Autodesk Inventor part; units mm, degrees
ref_plane "YZ Plane" through (0, 0, 0) normal (1, 0, 0) x (0, 1, 0)
ref_plane "XZ Plane" through (0, 0, 0) normal (0, 1, 0) x (-1, 0, 0)
ref_plane "XY Plane" through (0, 0, 0) normal (0, 0, 1) x (1, 0, 0)
sketch "Sketch2" plane through (0, 0, 0) normal (1, 0, 0) x (0, 1, 0)
  line L0 (0, 0) -> (39, 0)
  line L1 (44, -5) -> (44, -5)
  line L2 (34, -5) -> (0, -5)
  line L3 (0, -5) -> (0, 0)
  line L4 (39, -10) -> (39, -43)
  line L5 (44, -48) -> (44, -5)
  line L6 (0, -53) -> (0, -48)
  line L7 (39, -53) -> (0, -53)
  line L8 (0, -53) -> (0, -48)
  line L9 (0, -48) -> (34, -48)
  arc A0 (44, -5) -> (39, 0) centre (39, -5) ccw
  arc A1 (34, -48) -> (39, -43) centre (34, -43) ccw
  arc A2 (39, -10) -> (34, -5) centre (34, -10) ccw
  arc A3 (39, -53) -> (44, -48) centre (39, -48) ccw
  point P0 (44, 0)
  point P1 (0, -2.5)
  point P2 (0, -53)
  dimension "d12" = 44
  dimension "d14" = 5
  dimension "d17" = 5
  dimension "d18" = 39
  dimension "d19" = 5
  dimension "d42" = 43
extrude "Extrusion2" add sketch "Sketch2" along normal blind 14.25
fillet "Fillet1" radius 4 4 edges at (14.25, 0, -2.5) (0, 0, -2.5) (14.25, 0, -50.5) (0, 0, -50.5)
sketch "Sketch3" plane through (0, 39, 0) normal (0, 0, 1) x (1, 0, 0)
  circle A0 centre (7.125, -33.3) radius 2.8
  line L0 (0, 0) -> (0, -35)
  line L1 (4, -39) -> (10.25, -39)
  point P0 (0, -39)
  point P1 (7.125, -39)
  dimension "d23" = 5.6
  dimension "d24" = 7.125
  dimension "d25" = 5.7
extrude "Extrusion3" cut sketch "Sketch3" against normal blind 11.4
sketch "Sketch7" plane through (0, 39, -43) normal (0, -1, 0) x (1, 0, 0)
  circle A0 centre (7.125, 27) radius 1.5
  circle A1 centre (7.125, 6) radius 1.5
  line L0 (0, 33) -> (0, 0)
  line L1 (14.25, 33) -> (14.25, 0)
  line L2 (0, 33) -> (14.25, 33)
  line L3 (0, 0) -> (14.25, 0)
  circle A2 centre (7.125, 27) radius 2.8
  circle A3 centre (7.125, 6) radius 2.8
  point P0 (0, 43)
  dimension "d30" = 3
  dimension "d31" = 3
  dimension "d32" = 7.125
  dimension "d33" = 7.125
  dimension "d34" = 6
  dimension "d35" = 6
  dimension "d36" = 5.6
  dimension "d37" = 5.6
extrude "Extrusion5" cut sketch "Sketch7" against normal blind 8 contours A0 | A1
extrude "Extrusion6" cut sketch "Sketch7" against normal blind 2 contours A2 | A3
sketch "Sketch8" plane through (0, 34, -48) normal (0, 0, 1) x (1, 0, 0)
  circle A0 centre (7.125, -28.3) radius 2.8
  circle A1 centre (7.125, -28.3) radius 2.8
  point P0 (0, -34)
extrude "Extrusion7" add sketch "Sketch8" along normal blind 2
sketch "Sketch9" plane through (0, 44, -5) normal (0, 1, 0) x (1, 0, 0)
  circle A0 centre (7.125, 11) radius 1.5
  circle A1 centre (7.125, 11) radius 3.75
  line L0 (0, 43) -> (0, 0)
  line L1 (0, 21.5) -> (1.5875, 21.5)
  circle A2 centre (7.125, 32) radius 3.75
  point P0 (0, -5)
  dimension "d46" = 7.5
extrude "Extrusion8" cut sketch "Sketch9" against normal blind 2 contours A0 | A1 | A2
sketch "Sketch10" plane through (0, 44, -5) normal (0, 1, 0) x (1, 0, 0)
  line L0 (2.125, 17.5) -> (12.125, 17.5)
  line L1 (12.125, 17.5) -> (12.125, 25.5)
  line L2 (12.125, 25.5) -> (2.125, 25.5)
  line L3 (2.125, 25.5) -> (2.125, 17.5)
  line L4 (0, 43) -> (0, 0)
  line L5 (14.25, 43) -> (14.25, 0)
  line L6 (0, 0) -> (14.25, 0)
  point P0 (0, -5)
  point P1 (0, 21.5)
  point P2 (14.25, 21.5)
  dimension "d49" = 10
  dimension "d50" = 8
  dimension "d51" = 2.125
  dimension "d52" = 2.125
  dimension "d53" = 17.5
extrude "Extrusion9" cut sketch "Sketch10" against normal blind 50
fillet "Fillet2" radius 3 4 edges at (2.125, 41.5, -22.5) (2.125, 41.5, -30.5) (12.125, 41.5, -22.5) (12.125, 41.5, -30.5)
properties part number "ruka_part spodni"
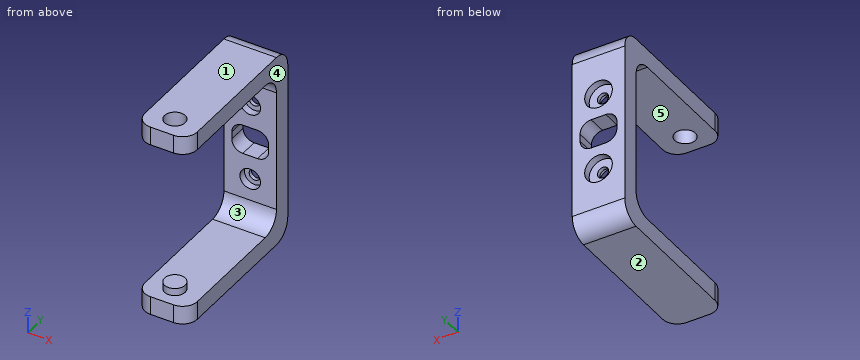
Design review of the part built by this model. Coordinates are the model's own, in mm. Face numbers are marked on the shaded views. A direction names the side the tool comes from. Coordinates: 2 decimals unless noted, no trailing zeros. Order: outer loops, then holes, each group sorted by start corner. A loop starts at its lowest first (then second) coordinate and runs counter-clockwise, first axis right, second up.
Item 1: For line 1 (X direction, y = 43.3, z = -37) (3 decimals); line 2 (Z direction, x = 3, y = 14); line 3 (Z direction, x = 5, y = 42.5), list the stretches that pass through material, from the lowest coordinate up.
Item 2: For the marked faces 4 and 5, list the 3-axis set-ups (+Z, -Z, +X, -X, +Y, -Y) from which the entire face can be reached by the end or side of a thin tool; tool diameter is ignored.
Item 3: The part is to be moulded in two halves that separate along Z. For the marked faces 1, 2 and 3, say which applies: pulls with the +Z half, pulls with the -Z half, needs draft (parallel to the pull), parting line crosses it, or undercut.
Item 4: Take a section at B-B, the plane z = -16. Write out the cut boundary in (x, y) (3 decimals).
Item 5: Take a section at C-C, the plane z = -3. Write out the cut boundary in (x, y) (3 decimals), then the cut area to 3 significant figures.
Item 6: Take a section at A-A, the plane y = 10. Write out the cut boundary in (x, z).
Item 7: For pin 1 Ø1.7 at (x, y) = (8.5, 6.5) entering from +Z; pin 2 Ø5 at (x, z) = (7.125, -16) entering from +Y; pin 3 Ø1.7 at (x, z) = (6, -16) entering from -Y; pin 4 Ø7 at (x, y) = (4.5, 8.5) entering from +Z, all flat-tipped, find the tip position at first contact; note any pin that passes through.
The answers:
1. line 1: x = 0 to 3.375, 10.875 to 14.25
1. line 2: z = -53 to -48, -5 to 0
1. line 3: z = -51.57 to -40.09, -33.91 to -30.5, -22.5 to -19.09, -12.91 to -1.43
2. face 4: +Z, -Z, +X, +Y, -Y
2. face 5: +X, -X, -Y
3. face 1: pulls with the +Z half
3. face 2: pulls with the -Z half
3. face 3: undercut
4. outline: (0, 39) - (4.325, 39) - (4.325, 41) - (5.625, 41) - (5.625, 42) - (3.375, 42) - (3.375, 44) - (0, 44) - close; (8.625, 41) - (9.925, 41) - (9.925, 39) - (14.25, 39) - (14.25, 44) - (10.875, 44) - (10.875, 42) - (8.625, 42) - close
5. outline: (0, 4) arc R4 ccw to (4, 0) - (10.25, 0) arc R4 ccw to (14.25, 4) - (14.25, 43.583) - (0, 43.583) - close; hole circle Ø5.6 at (7.125, 5.7)
5. area: 590 mm2
6. outline: (0, -53) - (14.25, -53) - (14.25, -48) - (0, -48) - close; (0, -5) - (14.25, -5) - (14.25, 0) - (0, 0) - close
7. pin 1: stops at z = -46
7. pin 2: stops at y = 42
7. pin 3: stops at y = 41
7. pin 4: stops at z = 0
